Input: part model. Units: mm. Frame: model coordinates. A direction names the side the tool comes from. Round coordinates to 2 decimals unless told otherwise and drop trailing zeros. Order: outer loops, then holes, each group sorted by start corner. A loop starts at its lowest first (then second) coordinate and runs counter-clockwise, first axis right, second up. Notation, with made-up numbers: (38, -37) - (73, -37) arc R29 cw to (73, -16) - close; hole circle Ø3 at (63.5, 21.25). An arc over 180 degrees is marked (long way). One line per item, written item: value. Start each with the question number.
from build123d import *

# Parameters (mm, degrees)
CROQUIS1_W              = 800
CROQUIS1_H              = 120
SALIENTE_EXTRUIR1_DEPTH = 300
CORTAR_EXTRUIR1_DEPTH   = 857.504524215
CORTAR_EXTRUIR2_DEPTH   = 600


with BuildPart() as part:
    # Croquis1 → Saliente-Extruir1 (new, symmetric)
    with BuildSketch(Plane.XY):
        Rectangle(CROQUIS1_W, CROQUIS1_H)
    extrude(amount=SALIENTE_EXTRUIR1_DEPTH, both=True)

    # Croquis2 → Cortar-Extruir1 (cut, through all)
    with BuildSketch(Plane(origin=(400, 0, 0), x_dir=(0, 0, -1), z_dir=(1, 0, 0))):
        Polygon((-208.038475773, 30), (-260, -60), (0, -60), (0, 30), align=None)
        Polygon((0, 30), (0, -60), (260, -60), (208.038475773, 30), align=None)
    extrude(amount=-CORTAR_EXTRUIR1_DEPTH, mode=Mode.SUBTRACT)

    # Croquis3 → Cortar-Extruir2 (cut)
    with BuildSketch(Plane.XY.offset(300)):
        Polygon((-324.585481157, 10), (-365, -60), (0, -60), (0, 10), align=None)
        Polygon((0, 10), (0, -60), (365, -60), (324.585481157, 10), align=None)
    extrude(amount=-CORTAR_EXTRUIR2_DEPTH, mode=Mode.SUBTRACT)


solid = part.part
1. Section A-A (y = -26.5). Return the cut outline in (x, z), then the cut area to 3 significant figures.
2. Section C-C (y = 21). Return the cut outline in (x, z), then the cut area to 3 significant figures.
3. Section D-D (z = 13.5). Return the cut outline in (x, y).
4. Set-up query: faces 4 (the face through (5, 10, 260)), 5 (the face through (1.867, 18.123, -214.895)), 6 (the face through (382, -60, -280)). Return all of +Z, -Z, +X, -X, +Y, -Y with unobstructed straight access to the full face (end or side cutting, diameter ignored); none if empty.
5. Pin query (flat end, axial travel): pin 1 (2 mm diameter, centred on x = 93.5, z = 85.5, fed in from -Y); pin 2 (24 mm diameter, centred on x = -24.5, z = 270.5, fed in from -Y). Return the tip coordinate at first contact, or that it passes through.
6. Pull-direction query (Z, two-part tool) for faces 1 (the face through (345.076, -25.49, 269.291)), 2 (the face through (31.5, 11.88, 218.5)), 3 (the face through (-6, 28, 300)); classes: released by +Z, released by -Z, zero draft, split by the parting line, or undercut.
7. Section B-B (x = 10.5). Return the cut outline in (y, z), then the cut area to 3 significant figures.
8. Line query: line 1 (Y direction, x = 156, z = 72); line 2 (Y direction, x = 239.5, z = 273.5); line 3 (X direction, y = 8.5, z = 257). Output: solid intervals per line, ascending. Write a range as from..to.
Solved:
1. outline: (-400, -300) - (-345.66, -300) - (-345.66, -240.66) - (-400, -240.66) - close; (-400, 240.66) - (-345.66, 240.66) - (-345.66, 300) - (-400, 300) - close; (345.66, -300) - (400, -300) - (400, -240.66) - (345.66, -240.66) - close; (345.66, 240.66) - (400, 240.66) - (400, 300) - (345.66, 300) - close
1. area: 12,900 mm²
2. outline: (-400, -300) - (400, -300) - (400, -213.23) - (-400, -213.23) - close; (-400, 213.23) - (400, 213.23) - (400, 300) - (-400, 300) - close
2. area: 139,000 mm²
3. outline: (-400, 30) - (400, 30) - (400, 60) - (-400, 60) - close
4. face 4: +Z, -Z, -Y
4. face 5: +X, -X, -Y
4. face 6: +Z, -Z, +X, -X, -Y
5. pin 1: stops at y = 30
5. pin 2: stops at y = 10
6. face 1: zero draft
6. face 2: undercut
6. face 3: released by +Z
7. outline: (10, -300) - (60, -300) - (60, 300) - (10, 300) - (10, 219.59) - (30, 208.04) - (30, -208.04) - (10, -219.59) - close
7. area: 21,400 mm²
8. line 1: y = 30..60
8. line 2: y = 10..60
8. line 3: x = -400..-325.45, 325.45..400
